Part print with two shaded views. Sizes in mm from the minimum x, y, z corner. A direction names the side the tool comes from. Give positions to 0.01 mm unless a question says otherwise; leave off trailing zeros. Loops run counter-clockwise (first coordinate to the right, second up) from the corner with the lowest first, then second, coordinate; pieces in that order, holes last. Notation, with made-up numbers: M 16.25,-7.75 L 22.25,-7.75 A23 cw 22.25,23.25 Z; hole C 25.25,85 d6. An arc over 180 degrees is marked long. Answer in a Markdown table with one row per item.
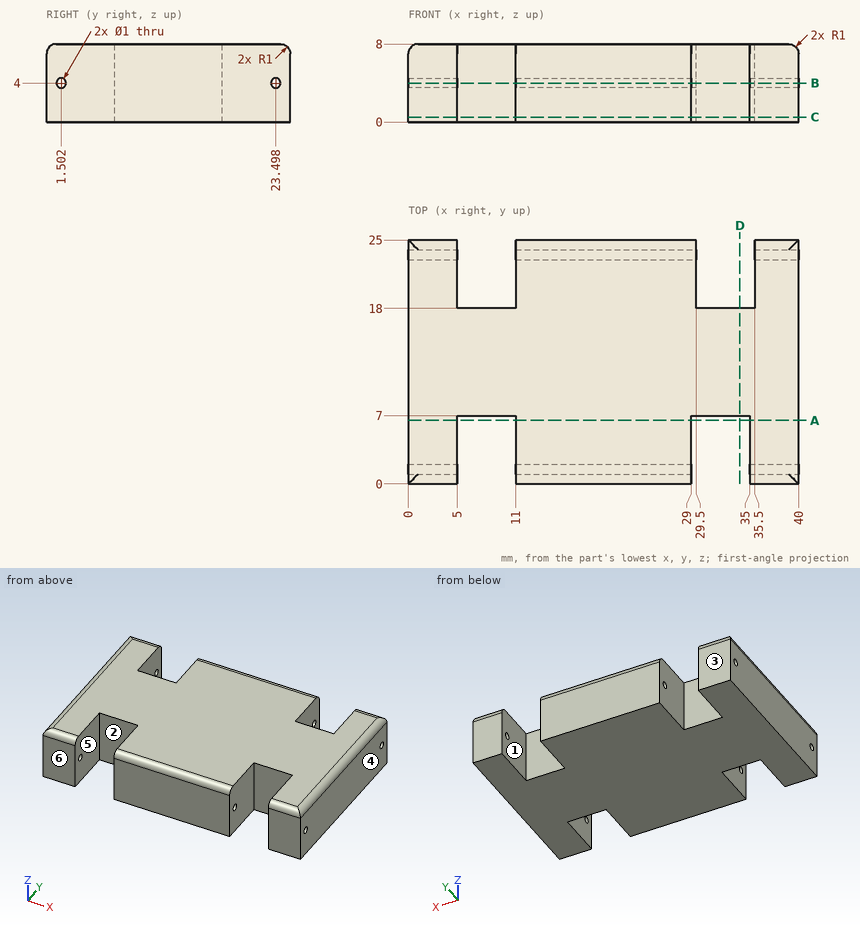
Q1. Saw through at A-A (y = 6.5). Give the cut face in (x, z), and give its area (3 significant figures).
Reported:
| item | result |
|---|---|
| outline | M 0,0 L 5,0 L 5,8 L 1,8 A1 ccw 0,7 Z; M 11,0 L 29,0 L 29,8 L 11,8 Z; M 35,0 L 40,0 L 40,7 A1 ccw 39,8 L 35,8 Z |
| area | 224 mm² |
Q2. Saw through at D-D (x = 34). Give the cut face in (y, z).
Reported:
| item | result |
|---|---|
| outline | M 7,0 L 18,0 L 18,8 L 7,8 Z |
Q3. Saw through at B-B (z = 4). Give the number of separate pieces and of enclosed holes in the cut face, and give its area (3 significant figures).
Reported:
| item | result |
|---|---|
| separate pieces | 7 |
| enclosed holes | 0 |
| area | 776 mm² |
Q4. 3-axis set-ups, long thin cutter, end or side, ignore diameter. For the marked faces 1, 2 and 3: which of +Z, -Z, +X, -X, +Y, -Y reach the whole face in a straight line?
Reported:
| item | result |
|---|---|
| face 1 | +Z, -Z, +Y |
| face 2 | +Z, -Z, -Y |
| face 3 | +Z, -Z, +X, -X, +Y |
Q5. Mould opens along X. For the marked faces 4, 5 and 6 say: released by +X, released by -X, zero draft, split by the parting line, or undercut.
Reported:
| item | result |
|---|---|
| face 4 | released by +X |
| face 5 | undercut |
| face 6 | zero draft |
Q6. Probe probe 1 along Y at (x, z) = (38.9, 4); probe 2 along X at (y, z) = (21.25, 2.5); probe 3 along X at (y, z) = (3.5, 7.5) (1 decimal). List the from-to ranges inside material, lowest first.
Reported:
| item | result |
|---|---|
| probe 1 | 0 to 1, 2 to 23, 24 to 25 |
| probe 2 | 0 to 5, 11 to 29.5, 35.5 to 40 |
| probe 3 | 0.1 to 5, 11 to 29, 35 to 39.9 |
Q7. Saw through at C-C (z = 0.5). Give the cut face in (x, y).
Reported:
| item | result |
|---|---|
| outline | M 0,0 L 5,0 L 5,7 L 11,7 L 11,0 L 29,0 L 29,7 L 35,7 L 35,0 L 40,0 L 40,25 L 35.5,25 L 35.5,18 L 29.5,18 L 29.5,25 L 11,25 L 11,18 L 5,18 L 5,25 L 0,25 Z |
Q8. Drop flat-ended pins along their axis: pin 1 (4 mm diameter, centred on x = 28, y = 5.5, fed in from -Z); pin 2 (1.5 mm diameter, centred on x = 32.5, z = 4, fed in from -Y). Give the stop position or say it passes through.
Reported:
| item | result |
|---|---|
| pin 1 | z = 0 |
| pin 2 | y = 7 |
